Geometry check sheet. Reference: the model listing, model coordinates, mm. A direction names the side the tool comes from. Coordinates: 2 decimals unless noted, no trailing zeros.
from build123d import *

# Parameters (mm, degrees)
SKETCH_1_R          = 1
SKETCH_1_W          = 124
SKETCH_1_H          = 82
EXTRUDE_2_DEPTH     = 20
SKETCH_2_W          = 127
SKETCH_2_H          = 85
CUT_EXTRUDE_1_DEPTH = 5
SKETCH_3_W          = 84.949028024
SKETCH_3_H          = 2
CUT_EXTRUDE_3_DEPTH = 164


with BuildPart() as part:
    # Эскиз1 → Бобышка-Вытянуть2 (new body)
    with BuildSketch(Plane(origin=(0, 0, 0), x_dir=(1, 0, 0), z_dir=(0, 1, 0))):
        with BuildLine():
            Line((3, 0), (127, 0))
            ThreePointArc((127, 0), (129.121320344, 0.878679656), (130, 3))
            Line((130, 3), (130, 85))
            ThreePointArc((130, 85), (129.121320344, 87.121320344), (127, 88))
            Line((127, 88), (3, 88))
            ThreePointArc((3, 88), (0.878679656, 87.121320344), (0, 85))
            Line((0, 85), (0, 3))
            ThreePointArc((0, 3), (0.878679656, 0.878679656), (3, 0))
        make_face()
        with Locations((120, 86.5)):
            Circle(SKETCH_1_R, mode=Mode.SUBTRACT)
        with Locations((10, 1.5)):
            Circle(SKETCH_1_R, mode=Mode.SUBTRACT)
        with Locations((65, 44)):
            Rectangle(SKETCH_1_W, SKETCH_1_H, mode=Mode.SUBTRACT)
    extrude(amount=EXTRUDE_2_DEPTH)

    # Эскиз2 → Вырез-Вытянуть1 (cut)
    with BuildSketch(Plane(origin=(0, 0, 0), x_dir=(-1, 0, 0), z_dir=(0, -1, 0))):
        with Locations((-65, 44)):
            Rectangle(SKETCH_2_W, SKETCH_2_H)
    extrude(amount=-CUT_EXTRUDE_1_DEPTH, mode=Mode.SUBTRACT)

    # Эскиз3 → Вырез-Вытянуть3 (cut)
    with BuildSketch(Plane.ZY):
        with Locations((-43.966717109, 3.987675958)):
            Rectangle(SKETCH_3_W, SKETCH_3_H)
    extrude(amount=-CUT_EXTRUDE_3_DEPTH, mode=Mode.SUBTRACT)


solid = part.part
1) Section check A-A on z = -48.5. Count the separate pieces of the cut face and the enclosed holes in it, and give its area (3 significant figures).
Data:
separate pieces: 4
enclosed holes: 0
area: 99.0 mm2
2) Access from +Z, -Z, +X, -X, +Y, -Y to the whole of each face (thin tool, end or side, straight path). Record for faces 5 (the flat face through (64, 12, -85)), 6 (the flat face through (1, 2.988, -44)), 7 (the flat face through (1.5, 1, -43)).
Data:
face 5: +Y, -Y
face 6: +X, -X
face 7: -Y
3) Depth check by flat-ended pin: pin 1 (1.6 mm diameter, centred on x = 10, z = -1.5, fed in from +Y); pin 2 (5.5 mm diameter, centred on y = 3.5, z = -63.5, fed in from -X); pin 3 (1.2 mm diameter, centred on x = 1, y = 4, fed in from +Z). Enter the tip coordinate at first touch or a pass-through.
Data:
pin 1: passes through
pin 2: stops at x = 0
pin 3: stops at z = -0.35
4) Mould release check, pull along X, two halves, no side actions. Record for faces 1 (the flat face through (64, 12, -3)), 2 (the flat face through (64, 10, 0)), 3 (the cylindrical face through (129.1, 9.86, -0.86)), 4 (the flat face through (128.5, 1, -43)): +X half, -X half, draft (parallel to the pull), parting line (faces both ways), or undercut.
Data:
face 1: undercut
face 2: draft
face 3: +X half
face 4: undercut
5) Material ranges on probe 1 along Z at (x, y) = (10, 15.25); probe 2 along Z at (x, y) = (10, 4.75); probe 3 along Z at (x, y) = (120, 10.5), recorded low to high.
Data:
probe 1: z = -88 to -85, -3 to -2.5, -0.5 to 0
probe 2: z = -88 to -86.5, -0.5 to 0
probe 3: z = -88 to -87.5, -85.5 to -85, -3 to 0
